Input: part model. Units: mm. Frame: model coordinates. A direction names the side the tool comes from. Coordinates: 2 decimals unless noted, no trailing zeros. Write each loop counter-clockwise with the first axis right and the second up, starting at its lowest first coordinate (ties: lowest second). Pieces come first, ordered by that corner, then holes. Notation, with made-up numbers: M 4.5,-13.75 L 40.5,-13.75 A22 cw 40.5,19.25 Z; hole C 82,5.5 d3. An arc over 180 degrees is marked long. Use CSV: the item, a comma, the result in double quotes.
```python
from build123d import *

# Parameters (mm, degrees)
F_1_2_0_5_DIAMETER_HOLE1_D           = 12.7
F_1_2_0_5_DIAMETER_HOLE1_DEPTH       = 38
F_1_2_0_5_DIAMETER_HOLE1_CSINK_D     = 13.97
F_1_2_0_5_DIAMETER_HOLE1_CSINK_ANGLE = 90
F_1_2_0_5_DIAMETER_HOLE1_TIP         = 3.815464931
FILLET1_R                            = 0.5
CUT_EXTRUDE2_DEPTH                   = 22
FILLET2_R                            = 1.5875
CHAMFER2_SIZE                        = 0.5
M8X1_25_TAPPED_HOLE1_D               = 6.8
M8X1_25_TAPPED_HOLE1_DEPTH           = 30
M8X1_25_TAPPED_HOLE1_TIP             = 2.042926105
CUT_EXTRUDE3_REACH                   = 131.151
CUT_EXTRUDE3_END_RADIUS              = 6.35
SKETCH9_W                            = 29.7
SKETCH9_H                            = 3.175
FILLET4_R                            = 1.5875


with BuildPart() as part:
    # Sketch1 → Revolve1 (revolve)
    with BuildSketch(Plane.XY, mode=Mode.PRIVATE) as revolve1_sk:
        Polygon((0, 0), (0, 10), (23.92, 10), (23.92, 9.5), (25.22, 9.5), (25.22, 10), (70.01, 10), (70.01, 9.5), (71.31, 9.5), (71.31, 10), (122.56, 10), (122.56, 12.5), (126.56, 12.5), (126.56, 9), (125.06, 9), (125.06, 6.375), (125.06, 0), (87.56, 0), align=None)
    revolve(revolve1_sk.sketch.rotate(Axis((-9.141012775, 0, 0), (1, 0, 0)), 90), axis=Axis((-9.141012775, 0, 0), (1, 0, 0)))

    # 1/2 (0.5) Diameter Hole1
    with Locations(Plane(origin=(125.06, 0, 0), x_dir=(0, 0, -1), z_dir=(1, 0, 0))):
        with Locations((0, 0)):
            CounterSinkHole(F_1_2_0_5_DIAMETER_HOLE1_D / 2, F_1_2_0_5_DIAMETER_HOLE1_CSINK_D / 2, depth=F_1_2_0_5_DIAMETER_HOLE1_DEPTH, counter_sink_angle=F_1_2_0_5_DIAMETER_HOLE1_CSINK_ANGLE)
            with Locations((0, 0, -(F_1_2_0_5_DIAMETER_HOLE1_DEPTH + F_1_2_0_5_DIAMETER_HOLE1_TIP / 2))):  # 118° drill point
                Cone(0, F_1_2_0_5_DIAMETER_HOLE1_D / 2, F_1_2_0_5_DIAMETER_HOLE1_TIP, mode=Mode.SUBTRACT)

    # Fillet1
    fillet1_edges = [part.edges().sort_by_distance(p)[0] for p in [
        (122.56, 0, -10),
    ]]
    fillet(fillet1_edges, radius=FILLET1_R)

    # Sketch6 → Cut-Extrude2 (cut)
    with BuildSketch(Plane.ZY):
        Polygon((-3, 73.427602241), (-3, 9.539392014), (-3, 7), (3, 7), (3, 9.539392014), (3, 73.427602241), (3, 201.204022694), (-3, 201.204022694), align=None)
    extrude(amount=-CUT_EXTRUDE2_DEPTH, mode=Mode.SUBTRACT)

    # Fillet2
    fillet2_edges = [part.edges().sort_by_distance(p)[0] for p in [
        (22, 8.269696007, -3),
        (22, 8.269696007, 3),
    ]]
    fillet(fillet2_edges, radius=FILLET2_R)

    # Chamfer2
    chamfer2_edges = [part.edges().sort_by_distance(p)[0] for p in [
        (0, -8.062257748, -5.916079783),
    ]]
    chamfer(chamfer2_edges, length=CHAMFER2_SIZE)

    # M8x1.25 Tapped Hole1
    with Locations(Plane.ZY):
        with Locations((0, 0)):
            Hole(M8X1_25_TAPPED_HOLE1_D / 2, depth=M8X1_25_TAPPED_HOLE1_DEPTH)
            with Locations((0, 0, -(M8X1_25_TAPPED_HOLE1_DEPTH + M8X1_25_TAPPED_HOLE1_TIP / 2))):  # 118° drill point
                Cone(0, M8X1_25_TAPPED_HOLE1_D / 2, M8X1_25_TAPPED_HOLE1_TIP, mode=Mode.SUBTRACT)

    # Cut-Extrude3: up to this cylinder (the profile starts outside it)
    cut_extrude3_end = Plane(origin=(106.91, 0, 0), z_dir=(1, 0, 0)) * Cylinder(CUT_EXTRUDE3_END_RADIUS, 276.002, mode=Mode.PRIVATE)
    # Sketch9 → Cut-Extrude3 (cut, up to the surface)
    with BuildSketch(Plane(origin=(0, 10, 0), x_dir=(1, 0, 0), z_dir=(0, 1, 0)), mode=Mode.PRIVATE) as cut_extrude3_sk1:
        with Locations((106.91, 0)):
            Rectangle(SKETCH9_W, SKETCH9_H)
    cut_extrude3_tool1 = extrude(cut_extrude3_sk1.sketch, amount=-CUT_EXTRUDE3_REACH, mode=Mode.PRIVATE) - cut_extrude3_end
    add(cut_extrude3_tool1.solids().sort_by_distance((106.91, 10, 0))[0], mode=Mode.SUBTRACT)

    # Fillet4
    fillet4_edges = [part.edges().sort_by_distance(p)[0] for p in [
        (92.06, 8.010774594, 1.5875),
        (121.76, 8.010774594, 1.5875),
        (121.76, 8.010774594, -1.5875),
        (92.06, 8.010774594, -1.5875),
    ]]
    fillet(fillet4_edges, radius=FILLET4_R - 0.0001)  # a hair under: the kernel refuses the full size


solid = part.part
```
1. Mould query, pull axis X, two halves, no side actions, for faces 1 (the flat face through (25.22, 4, -9)), 2 (the flat face through (0, -4, 0)), 3 (the flat face through (126.56, -3, -9)), 4 (the cylindrical face through (125.8, -6.083, -6.633)). Classes: pulls with the +X half, pulls with the -X half, needs draft (parallel to the pull), parting line crosses it, or undercut.
Resolved:
face 1,"undercut"
face 2,"pulls with the -X half"
face 3,"pulls with the +X half"
face 4,"needs draft"
2. Section B-B (x = 109). Return loops of the section in (y, z).
Resolved:
outline,"M 6.15,-1.59 A6.35 cw long 6.15,1.59 L 9.87,1.59 A10 ccw long 9.87,-1.59 Z"
3. Section A-A (x = 90.5). Return loops of the section in (y, z).
Resolved:
outline,"C 0,0 d20; hole C 0,0 d12.7"
4. Access query for faces 5 (the cylindrical face through (70.669, 9.274, -2.059)), 6 (the flat face through (22, 9, 0)), 7 (the cylindrical face through (97, 0, -10)), 8 (the flat face through (107, 8, -1.588)). Directions: +Z, -Z, +X, -X, +Y, -Y. A direction counts if a zero-diameter tool reaches every point of the face in a straight line with its end or side. Return the directions, or none.
Resolved:
face 5,"none"
face 6,"-X, +Y"
face 7,"-X"
face 8,"+Y"
5. Contact query for flat-ended pins moving along their axis: pin 1 Ø1.5 at (y, z) = (2, -2) entering from +X; pin 2 Ø2 at (x, y) = (27.5, 3.5) entering from +Z; pin 3 Ø2 at (x, y) = (35.5, -10) entering from +Z. Output: stop coordinate, or through.
Resolved:
pin 1,"stops at x = 85.39"
pin 2,"stops at z = 9.68"
pin 3,"stops at z = 4.36"
6. Material intervals for line 1 (X direction, y = 7.75, z = 0); line 2 (Y direction, x = 8.75, z = 0); line 3 (Y direction, x = 107.5, z = 0), sorted ascending. Write a range as [from, to].
Resolved:
line 1,"x = [22, 92.06], [121.76, 125.06]"
line 2,"y = [-10, -3.4], [3.4, 7]"
line 3,"y = [-10, -6.35]"
